Source: CAD feature listing. Evaluate the final solid. Frame: model axes, mm. A direction names the side the tool comes from. Give positions to 0.01 mm unless a question says otherwise; leave off trailing zeros. Loops run counter-clockwise (first coordinate to the right, second up) from the corner with the lowest first, then second, coordinate; pieces in that order, holes last. Notation, with made-up numbers: (78, 49) -> (137, 49) arc R22 ccw to (137, 82) -> close; hole circle Ø8 at (-35.5, 27). An arc over 180 degrees is marked (long way). Answer as a JSON object with one key per item and string values. Group by question number.
from build123d import *

# Parameters (mm, degrees)
SKETCH1_R                                            = 15.5
SKETCH1_R_2                                          = 1.5
SKETCH1_R_3                                          = 2.7
BOSS_EXTRUDE1_DEPTH                                  = 14.5
SKETCH2_W                                            = 42.2
SKETCH2_H                                            = 42.2
CUT_EXTRUDE1_DEPTH                                   = 4
SKETCH3_R                                            = 8
CUT_EXTRUDE2_DEPTH                                   = 5
FILLET2_R                                            = 10
TALADRO_DE_MARGEN_PARA_M31_D                         = 3.6
SKETCH7_R                                            = 1.5
CUT_EXTRUDE3_DEPTH                                   = 91.38445183
REFRENTADO_PARA_TORNILLO_CON_CABEZA_TRON_D           = 3.6
REFRENTADO_PARA_TORNILLO_CON_CABEZA_TRON_CBORE_D     = 7
REFRENTADO_PARA_TORNILLO_CON_CABEZA_TRON_CBORE_DEPTH = 4.4
FILLET3_R                                            = 5


with BuildPart() as part:
    # Sketch1 → Boss-Extrude1 (new body)
    with BuildSketch(Plane.XY):
        with BuildLine():
            Line((42.669600757, 14), (42.669600757, 21.1))
            Line((42.669600757, 21.1), (84.869600757, 21.1))
            Line((84.869600757, 21.1), (84.869600757, -21.1))
            Line((84.869600757, -21.1), (42.669600757, -21.1))
            Line((42.669600757, -21.1), (42.669600757, -14))
            Line((42.669600757, -14), (23.669600757, -14))
            ThreePointArc((23.669600757, -14), (-27.5, 0), (23.669600757, 14))
            Line((23.669600757, 14), (42.669600757, 14))
        make_face()
        with Locations(Location((63.769600757, 0, 0), (0, 0, 180))):
            Circle(SKETCH1_R, mode=Mode.SUBTRACT)
        with Locations(Location((48.269600757, 15.5, 0), (0, 0, 180))):
            Circle(SKETCH1_R_2, mode=Mode.SUBTRACT)
        with Locations(Location((79.269600757, 15.5, 0), (0, 0, 180))):
            Circle(SKETCH1_R_2, mode=Mode.SUBTRACT)
        with Locations(Location((79.269600757, -15.5, 0), (0, 0, 180))):
            Circle(SKETCH1_R_2, mode=Mode.SUBTRACT)
        with Locations(Location((48.269600757, -15.5, 0), (0, 0, 180))):
            Circle(SKETCH1_R_2, mode=Mode.SUBTRACT)
        with Locations(Location((0, 0, 0), (0, 0, 180))):
            Circle(SKETCH1_R_3, mode=Mode.SUBTRACT)
    extrude(amount=BOSS_EXTRUDE1_DEPTH)

    # Sketch2 → Cut-Extrude1 (cut)
    with BuildSketch(Plane(origin=(0, 0, 0), x_dir=(-1, 0, 0), z_dir=(0, 0, -1))):
        with Locations((-63.769600757, 0)):
            Rectangle(SKETCH2_W, SKETCH2_H)
    extrude(amount=-CUT_EXTRUDE1_DEPTH, mode=Mode.SUBTRACT)

    # Sketch3 → Cut-Extrude2 (cut)
    with BuildSketch(Plane.XY.offset(14.5)):
        Circle(SKETCH3_R)
    extrude(amount=-CUT_EXTRUDE2_DEPTH, mode=Mode.SUBTRACT)

    # Fillet2
    # the kernel refuses this fillet: 10 mm, written as the material it adds along each edge
    with BuildSketch(Plane(origin=(42.669600757, -14, 4), x_dir=(-1, 0, 0), z_dir=(0, 0, 1))) as fillet2_piece_1:
        with BuildLine():
            CenterArc((9.570266454, 10), FILLET2_R, 196.857956022, 73.142043978)
            Line((0, 7.1), (0, 0))
            Line((0, 0), (9.570266454, 0))
        make_face()
    extrude(amount=10.5)
    with BuildSketch(Plane(origin=(42.669600757, 14, 4), x_dir=(-1, 0, 0), z_dir=(0, 0, 1))) as fillet2_piece_2:
        with BuildLine():
            CenterArc((9.570266454, -10), FILLET2_R, 90, 73.142043978)
            Line((0, -7.1), (0, 0))
            Line((0, 0), (9.570266454, 0))
        make_face()
    extrude(amount=10.5)
    with BuildSketch(Plane(origin=(23.669600757, -14, 0), x_dir=(-0.5763974746684583, -0.8171694751982751, 0), z_dir=(0, 0, 1))) as fillet2_piece_3:
        with BuildLine():
            CenterArc((5.206441973, 9.967869045), FILLET2_R, 215.197557054, 50.2081805)
            Line((-2.965252779, 4.203894298), (0, 0))
            ThreePointArc((0, 0), (2.20272545, 0.088360126), (4.4054509, 0))
        make_face()
    extrude(amount=14.5)
    with BuildSketch(Plane(origin=(23.669600757, 14, 0), x_dir=(1, 0, 0), z_dir=(0, 0, 1))) as fillet2_piece_4:
        with BuildLine():
            CenterArc((5.144458311, 10), FILLET2_R, 219.7918195, 50.2081805)
            ThreePointArc((-2.539290774, 3.6), (-1.197440189, 1.850930553), (0, 0))
            Line((0, 0), (5.144458311, 0))
        make_face()
    extrude(amount=14.5)

    # Taladro de margen para M31 (through all)
    with Locations(Plane.XY.offset(14.5)):
        with Locations((79.269600757, -15.5), (79.269600757, 15.5), (48.269600757, 15.5), (48.269600757, -15.5)):
            Hole(TALADRO_DE_MARGEN_PARA_M31_D / 2)

    # Sketch7 → Cut-Extrude3 (cut, through all)
    with BuildSketch(Plane.XY.offset(14.5)):
        with Locations((34.956696686, 7)):
            Circle(SKETCH7_R)
        with Locations((34.956696686, -7)):
            Circle(SKETCH7_R)
    extrude(amount=-CUT_EXTRUDE3_DEPTH, mode=Mode.SUBTRACT)

    # Refrentado para tornillo con cabeza troncocónica de M31 (through all)
    with Locations(Plane.XY.offset(14.5)):
        with Locations((34.956696686, 7), (34.956696686, -7)):
            CounterBoreHole(REFRENTADO_PARA_TORNILLO_CON_CABEZA_TRON_D / 2, REFRENTADO_PARA_TORNILLO_CON_CABEZA_TRON_CBORE_D / 2, REFRENTADO_PARA_TORNILLO_CON_CABEZA_TRON_CBORE_DEPTH)

    # Fillet3
    fillet3_edges = [part.edges().sort_by_distance(p)[0] for p in [
        (84.869600757, -21.1, 9.25),
        (42.669600757, -21.1, 9.25),
        (42.669600757, 21.1, 9.25),
        (84.869600757, 21.1, 9.25),
    ]]
    fillet(fillet3_edges, radius=FILLET3_R)


solid = part.part
(1) Access query for faces 4 (the face through (-1.73, -7.81, 12.04)), 5 (the face through (38.03, -15.3, 9.18)), 6 (the face through (63, -21.1, 9)). Directions: +Z, -Z, +X, -X, +Y, -Y. A direction counts if a zero-diameter tool reaches every point of the face in a straight line with its end or side. Return the directions, or none.
(2) Section query A-A on x = 0. Return the cut outline in (y, z).
(3) First-contact query: pin 1 (4 mm diameter, centred on x = 33.5, z = 5, fed in from +Y); pin 2 (1 mm diameter, centred on x = 5, z = 4.5, fed in from +Y); pin 3 (6 mm diameter, centred on x = 0, y = 0, fed in from -Z); pin 4 (3 mm diameter, centred on x = 34.96, y = 7, fed in from +Z). Flat tips, straight axial feed; report the tip coordinate or a pass-through.
(4) Mould query, pull axis X, two halves, no side actions, for faces 1 (the face through (81, -15, 9)), 2 (the face through (29, 0, 14.5)), 3 (the face through (83, 20, 9)). Classes: pulls with the +X half, pulls with the -X half, needs draft (parallel to the pull), parting line crosses it, or undercut.
(5) Section query D-D on z = 11.75. State how many separate pieces and enclosed holes the cut face has, plus the area to 3 significant figures.
(6) Section query C-C on z = 1.25. Return the cut outline in (x, y), plus the area to 3 significant figures.
(7) Section query B-B on y = 0. Return the cut outline in (x, z), plus the area to 3 significant figures.
(8) Material intervals for line 1 (X direction, y = -1, z = 5); line 2 (Y direction, x = 69, z = 9.25); line 3 (Z direction, x = -2, y = -2), sorted ascending. Write a range as from..to.
Result:
{
 "1": {"face 4": "+Z", "face 5": "+Z, -Z, -Y", "face 6": "+Z, -Z, +X, -Y"},
 "2": {"outline": "(-27.5, 0) -> (-2.7, 0) -> (-2.7, 9.5) -> (-8, 9.5) -> (-8, 14.5) -> (-27.5, 14.5) -> close; (2.7, 0) -> (27.5, 0) -> (27.5, 14.5) -> (8, 14.5) -> (8, 9.5) -> (2.7, 9.5) -> close"},
 "3": {"pin 1": "y = 14.29", "pin 2": "y = 27.13", "pin 3": "z = 0", "pin 4": "through"},
 "4": {"face 1": "undercut", "face 2": "needs draft", "face 3": "pulls with the +X half"},
 "5": {"separate pieces": "1", "enclosed holes": "8", "area": "3,570 mm²"},
 "6": {"outline": "(21.13, -17.6) arc R10 cw to (28.81, -14) -> (42.67, -14) -> (42.67, 14) -> (28.81, 14) arc R10 cw to (21.13, 17.6) arc R27.5 ccw (long way) to start; hole circle Ø5.4 at (0, 0); hole circle Ø3.6 at (34.96, -7); hole circle Ø3.6 at (34.96, 7)", "area": "2,800 mm²"},
 "7": {"outline": "(-27.5, 0) -> (-2.7, 0) -> (-2.7, 9.5) -> (-8, 9.5) -> (-8, 14.5) -> (-27.5, 14.5) -> close; (2.7, 0) -> (42.67, 0) -> (42.67, 4) -> (48.27, 4) -> (48.27, 14.5) -> (8, 14.5) -> (8, 9.5) -> (2.7, 9.5) -> close; (79.27, 4) -> (84.87, 4) -> (84.87, 14.5) -> (79.27, 14.5) -> close", "area": "1,000 mm²"},
 "8": {"line 1": "-27.48..-2.51, 2.51..48.3, 79.24..84.87", "line 2": "-21.1..-14.59, 14.59..21.1", "line 3": "0..9.5"}
}
